Input: part model. Units: mm. Frame: model coordinates. A direction names the side the tool comes from. Round coordinates to 2 decimals unless told otherwise and drop trailing zeros. Order: outer loops, then holes, each group sorted by start corner. A loop starts at its lowest first (then second) coordinate and runs counter-clockwise, first axis right, second up. Notation, with made-up numbers: (76, 49.5) -> (117, 49.5) arc R20 cw to (117, 61.5) -> close; hole circle Ø6 at (30.5, -3.5). An arc over 180 degrees is marked (long way). Use a Markdown table: item, result.
from build123d import *

# Parameters (mm, degrees)
SKETCH1_W           = 45
SKETCH1_H           = 45
BOSS_EXTRUDE1_DEPTH = 25
SKETCH3_W           = 45
SKETCH3_H           = 10
BOSS_EXTRUDE2_DEPTH = 35
SKETCH4_R           = 5
CUT_EXTRUDE4_DEPTH  = 28.5
CUT_EXTRUDE5_DEPTH  = 46
FILLET1_R           = 10


with BuildPart() as part:
    # Sketch1 → Boss-Extrude1 (new body)
    with BuildSketch(Plane.XY):
        with Locations((22.5, 22.5)):
            Rectangle(SKETCH1_W, SKETCH1_H)
    extrude(amount=BOSS_EXTRUDE1_DEPTH)

    # Sketch3 → Boss-Extrude2 (add)
    with BuildSketch(Plane.XY.offset(25)):
        with Locations((22.5, 22.5)):
            Rectangle(SKETCH3_W, SKETCH3_H)
    extrude(amount=BOSS_EXTRUDE2_DEPTH)

    # Sketch4 → Cut-Extrude4 (cut, through all)
    with BuildSketch(Plane.XZ.offset(-17.5)):
        with Locations((22.5, 50.5)):
            Circle(SKETCH4_R)
        with BuildLine():
            ThreePointArc((33.245992167, 33.632171084), (34.776451354, 40.535626355), (27.872996083, 42.066085542))
            ThreePointArc((27.872996083, 42.066085542), (22.5, 40.5), (17.127003917, 42.066085542))
            ThreePointArc((17.127003917, 42.066085542), (10.223548646, 40.535626355), (11.754007833, 33.632171084))
            ThreePointArc((11.754007833, 33.632171084), (22.5, 30.5), (33.245992167, 33.632171084))
        make_face()
    extrude(amount=-CUT_EXTRUDE4_DEPTH, mode=Mode.SUBTRACT)

    # Sketch5 → Cut-Extrude5 (cut, through all)
    with BuildSketch(Plane(origin=(0, 0, 0), x_dir=(1, 0, 0), z_dir=(0, 1, 0))):
        Polygon((45, -25), (32.261041801, -60), (45, -60), align=None)
        Polygon((0, -25), (12.738958199, -60), (0, -60), align=None)
    extrude(amount=CUT_EXTRUDE5_DEPTH, mode=Mode.SUBTRACT)

    # Fillet1
    fillet1_edges = [part.edges().sort_by_distance(p)[0] for p in [
        (12.738958199, 22.5, 60),
        (32.261041801, 22.5, 60),
    ]]
    fillet(fillet1_edges, radius=FILLET1_R)


solid = part.part
1) Cut plane B-B on z = 50.5. Return loops of the section in (x, y).
Results found:
| item | result |
|---|---|
| outline | (9.28, 17.5) -> (17.5, 17.5) -> (17.5, 27.5) -> (9.28, 27.5) -> close; (27.5, 17.5) -> (35.72, 17.5) -> (35.72, 27.5) -> (27.5, 27.5) -> close |
2) Cut plane D-D on y = 31. Return loops of the section in (x, z).
Results found:
| item | result |
|---|---|
| outline | (0, 0) -> (45, 0) -> (45, 25) -> (0, 25) -> close |
3) Pin query (flat end, axial travel): pin 1 Ø17.5 at (x, z) = (26.5, 38.5) entering from -Y; pin 2 Ø1.5 at (x, y) = (25.5, 35) entering from +Z. Return the tip coordinate at first contact, or that it passes through.
Results found:
| item | result |
|---|---|
| pin 1 | stops at y = 17.5 |
| pin 2 | stops at z = 25 |
4) Cut plane A-A on x = 22.5. Return loops of the section in (y, z).
Results found:
| item | result |
|---|---|
| outline | (0, 0) -> (45, 0) -> (45, 25) -> (27.5, 25) -> (27.5, 30.5) -> (17.5, 30.5) -> (17.5, 25) -> (0, 25) -> close; (17.5, 40.5) -> (27.5, 40.5) -> (27.5, 45.5) -> (17.5, 45.5) -> close; (17.5, 55.5) -> (27.5, 55.5) -> (27.5, 60) -> (17.5, 60) -> close |
5) Pull-direction query (Z, two-part tool) for faces 4 (the flat face through (22, 27.5, 42)), 5 (the cylindrical face through (22.3, 22.4, 30.5)), 6 (the cylindrical face through (13.935, 22.57, 58.142)), 7 (the cylindrical face through (22.6, 22.4, 40.5)); classes: +Z half, -Z half, draft (parallel to the pull), parting line (faces both ways), or undercut.
Results found:
| item | result |
|---|---|
| face 4 | draft |
| face 5 | undercut |
| face 6 | +Z half |
| face 7 | undercut |
6) Cut plane C-C on x = 15.5. Return loops of the section in (y, z) (3 decimals), and give its area (3 significant figures).
Results found:
| item | result |
|---|---|
| outline | (0, 0) -> (45, 0) -> (45, 25) -> (27.5, 25) -> (27.5, 31.765) -> (17.5, 31.765) -> (17.5, 25) -> (0, 25) -> close; (17.5, 42.736) -> (27.5, 42.736) -> (27.5, 59.056) -> (17.5, 59.056) -> close |
| area | 1,360 mm² |
7) Set-up query: faces 1 (the flat face through (22, 17.5, 42)), 2 (the flat face through (22, 36, 25)), 3 (the flat face through (45, 22, 12)). Return all of +Z, -Z, +X, -X, +Y, -Y with unobstructed straight access to the full face (end or side cutting, diameter ignored); none if empty.
Results found:
| item | result |
|---|---|
| face 1 | +Z, +X, -X, -Y |
| face 2 | +Z, +X, -X, +Y |
| face 3 | +Z, -Z, +X, +Y, -Y |
8) Line query: L1, parallel to Z at x = 22.5, y = 23.25; L2, parallel to Z at x = 4.5, y = 6.5; L3, parallel to Y at x = 5, z = 33. Output: solid intervals per line, ascending. Write a range as [from, to].
Results found:
| item | result |
|---|---|
| L1 | z = [0, 30.5], [40.5, 45.5], [55.5, 60] |
| L2 | z = [0, 25] |
| L3 | y = [17.5, 27.5] |
